CAD build for the part. Positions are in the model's coordinates, mm. A direction names the side the tool comes from. Coordinates: 2 decimals unless noted, no trailing zeros. Order: outer loops, then holes, each group sorted by start corner. A loop starts at its lowest first (then second) coordinate and runs counter-clockwise, first axis right, second up. Notation, with made-up numbers: (77.25, -15.5) - (92.25, -15.5) arc R27 cw to (92.25, 17.5) - close; hole circle Ø8 at (39, -6). An arc over 180 degrees is marked (long way). Return JSON: item names as keys, results as strings.
from build123d import *

# Parameters (mm, degrees)
F0_R     = 69.85
F1_DEPTH = 19.05
F2_R     = 35.052
F3_DEPTH = 34.798
F4_R     = 19.05
F5_DEPTH = 53.849


with BuildPart() as f1:
    # F0 (on Front) → F1 (new body)
    with BuildSketch(Plane.XZ):
        with Locations((-39.630193, -28.484197)):
            Circle(F0_R)
    extrude(amount=F1_DEPTH)

    # F2 (on face) → F3 (join)
    with BuildSketch(Plane.XZ.offset(19.05)):
        with Locations((-39.630193, -28.484197)):
            Circle(F2_R)
    extrude(amount=F3_DEPTH)

    # F4 (on face) → F5 (cut, through all)
    with BuildSketch(Plane.XZ.offset(53.848)):
        with Locations((-39.630193, -28.484197)):
            Circle(F4_R)
    extrude(amount=-F5_DEPTH, mode=Mode.SUBTRACT)


solid = f1.part
Item 1: Wall check: L1, parallel to Y at x = -0.5, z = -49; L2, parallel to X at y = -6.5, z = -12.5; L3, parallel to X at y = -12, z = -70.5. Give the ranges that are in metal, low to high. Write a range as [from, to].
Findings below:
{"L1": "y = [-19.05, 0]", "L2": "x = [-107.63, -49.99], [-29.27, 28.37]", "L3": "x = [-95.43, 16.17]"}
Item 2: Drop flat-ended pins along their axis: P1, Ø1.5, axis at x = -18.5, y = -10, coming from the -Z side; P2, Ø5, axis at x = -57, y = -11, coming from the +Z side; P3, Ø5, axis at y = -6, z = -4, coming from the -X side. Give the stop position or say it passes through.
Findings below:
{"P1": "stops at z = -95.29", "P2": "stops at z = 39.76", "P3": "stops at x = -105.93"}
Item 3: Band-saw the part on B-B, the plane x = -40.5. List the corners of the cut face in (y, z), then the cut area to 3 significant figures.
Findings below:
{"outline": "(-53.85, -63.53) - (-19.05, -63.53) - (-19.05, -98.33) - (0, -98.33) - (0, -47.51) - (-53.85, -47.51) - close; (-53.85, -9.45) - (0, -9.45) - (0, 41.36) - (-19.05, 41.36) - (-19.05, 6.56) - (-53.85, 6.56) - close", "area": "3,050 mm²"}
Item 4: Mould opens along Z. For faces 1 (the cylindrical face through (-7.25, -36.21, -41.91)), 2 (the flat face through (-25, 0, -43)), 3 (the cylindrical face through (-58.66, -27.3, -27.65)) say: released by +Z, released by -Z, zero draft, split by the parting line, or undercut.
Findings below:
{"face 1": "split by the parting line", "face 2": "zero draft", "face 3": "undercut"}
Item 5: Which spindle directions (+Z, -Z, +X, -X, +Y, -Y) get a long thin tool onto all of the face, cutting with end or side? Do faces 4 (the cylindrical face through (24.893, -9.392, -55.237)), 5 (the flat face through (-25, -19.05, 4)). Say none if no direction does.
Findings below:
{"face 4": "+Y, -Y", "face 5": "-Y"}
Item 6: Band-saw the part on D-D, the plane y = -34.5. List the corners of the cut face in (x, z), then the cut area to 3 significant figures.
Findings below:
{"outline": "circle Ø70.1 at (-39.63, -28.48); hole circle Ø38.1 at (-39.63, -28.48)", "area": "2,720 mm²"}
Item 7: Band-saw the part on A-A, the plane z = -25. List the corners of the cut face in (x, y).
Findings below:
{"outline": "(-109.39, -19.05) - (-74.51, -19.05) - (-74.51, -53.85) - (-58.36, -53.85) - (-58.36, 0) - (-109.39, 0) - close; (-20.9, -53.85) - (-4.75, -53.85) - (-4.75, -19.05) - (30.13, -19.05) - (30.13, 0) - (-20.9, 0) - close"}
Item 8: Band-saw the part on C-C, the plane z = -55. List the corners of the cut face in (x, y).
Findings below:
{"outline": "(-104.25, -19.05) - (-62.56, -19.05) - (-62.56, -53.85) - (-16.71, -53.85) - (-16.71, -19.05) - (24.99, -19.05) - (24.99, 0) - (-104.25, 0) - close"}
